```python
from build123d import *

# Parameters (mm, degrees)
SKETCH1_W           = 64.2
SKETCH1_H           = 22.5
SKETCH1_R           = 1.5
BOSS_EXTRUDE1_DEPTH = 18.8
SKETCH2_R           = 3
BOSS_EXTRUDE2_DEPTH = 18.4
SKETCH3_W           = 2.4
SKETCH3_H           = 2.701398926
SKETCH3_R           = 0.7
BOSS_EXTRUDE3_DEPTH = 1
FILLET1_R           = 2


with BuildPart() as part:
    # Sketch1 → Boss-Extrude1 (new body)
    with BuildSketch(Plane(origin=(0, 0, 0), x_dir=(1, 0, 0), z_dir=(0, 1, 0))):
        with Locations((32.1, 11.25)):
            Rectangle(SKETCH1_W, SKETCH1_H)
        with Locations(Location((32.4, 2.25, 0), (0, 0, 270))):
            Circle(SKETCH1_R, mode=Mode.SUBTRACT)
        with Locations(Location((32.4, 20.25, 0), (0, 0, 90))):
            Circle(SKETCH1_R, mode=Mode.SUBTRACT)
    extrude(amount=BOSS_EXTRUDE1_DEPTH)

    # Sketch2 → Boss-Extrude2 (add, symmetric)
    with BuildSketch(Plane(origin=(0, 9, 0), x_dir=(1, 0, 0), z_dir=(0, 1, 0))):
        with Locations(Location((53, 11.25, 0), (0, 0, 90))):
            Circle(SKETCH2_R)
    extrude(amount=BOSS_EXTRUDE2_DEPTH, both=True)

    # Sketch3 → Boss-Extrude3 (add, symmetric)
    with BuildSketch(Plane(origin=(0, 9, 0), x_dir=(1, 0, 0), z_dir=(0, 1, 0))):
        with Locations((65.4, 11.25)):
            Rectangle(SKETCH3_W, SKETCH3_H)
        with Locations(Location((65.4, 11.25, 0), (0, 0, 270))):
            Circle(SKETCH3_R, mode=Mode.SUBTRACT)
    extrude(amount=BOSS_EXTRUDE3_DEPTH, both=True)

    # Fillet1
    fillet1_edges = [part.edges().sort_by_distance(p)[0] for p in [
        (64.2, 9.4, -22.5),
        (64.2, 9.4, 0),
    ]]
    fillet(fillet1_edges, radius=FILLET1_R)


solid = part.part
```
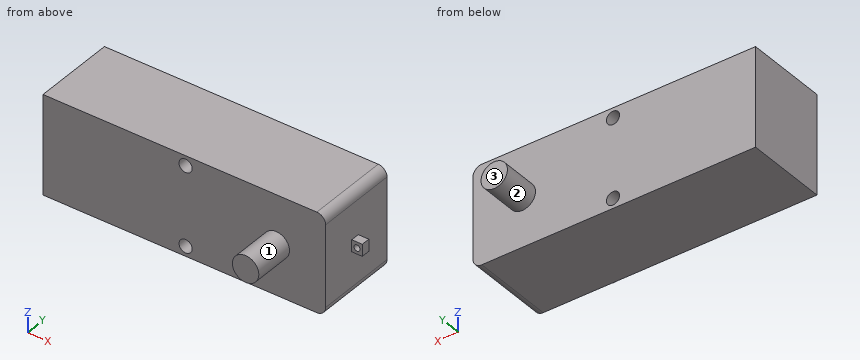
Could you check a few things on this model? Use its own coordinates, in mm. Face numbers are marked on the shaded views. A direction names the side the tool comes from. Round coordinates to 2 decimals unless told otherwise and drop trailing zeros. Loops run counter-clockwise (first coordinate to the right, second up) from the corner with the lowest first, then second, coordinate; pieces in that order, holes last. Notation, with made-up numbers: M 88.25,86.5 L 125.25,86.5 A12 cw 125.25,98.5 Z; hole C 19.25,-7.75 d11. An arc over 180 degrees is marked long. Put each result on its own line as item: value.
Q1. On a 3-axis mill with a long thin cutter (end or side, diameter ignored), from which of +Z, -Z, +X, -X, +Y, -Y can I reach the whole of each face in a straight line? I mean the marked faces 1, 2 and 3. Say none if no direction works.
Check result:
face 1: -Y
face 2: +Y
face 3: +Z, -Z, +X, -X, +Y
Q2. Imagine slicing it at C-C (y = 3). Write out the boundary of the cut face in (x, z).
Check result:
outline: M 0,-22.5 L 62.2,-22.5 A2 ccw 64.2,-20.5 L 64.2,-2 A2 ccw 62.2,0 L 0,0 Z; hole C 32.4,-20.25 d3; hole C 32.4,-2.25 d3
Q3. I need wall thicknesses on probe 1 along Z at (x, y) = (32.5, 12); probe 2 along X at (y, z) = (14.5, -2.25); probe 3 along Y at (x, z) = (19.5, -15.25). Which ranges of each line are inside material? Lowest first, please.
Check result:
probe 1: -22.5 to -21.75, -18.75 to -3.75, -0.75 to 0
probe 2: 0 to 30.9, 33.9 to 64.2
probe 3: 0 to 18.8
Q4. Imagine slicing it at B-B (z = -11.25). Write out the boundary of the cut face in (x, y).
Check result:
outline: M 0,0 L 50,0 L 50,-9.4 L 56,-9.4 L 56,0 L 64.2,0 L 64.2,8 L 64.7,8 L 64.7,10 L 64.2,10 L 64.2,18.8 L 56,18.8 L 56,27.4 L 50,27.4 L 50,18.8 L 0,18.8 Z; M 66.1,8 L 66.6,8 L 66.6,10 L 66.1,10 Z
Q5. For pin 1 (5 mm diameter, centred on x = 49.5, z = -5.5, fed in from -Y); pin 2 (11 mm diameter, centred on x = 19, z = -9.5, fed in from +Y); pin 3 (1.6 mm diameter, centred on x = 65.4, z = -11.25, fed in from -Y); pin 4 (1.8 mm diameter, centred on x = 32.4, z = -2.25, fed in from -Y), each with a flat end and sliding along its axis, tell me the tip position at first contact or that it passes through.
Check result:
pin 1: y = 0
pin 2: y = 18.8
pin 3: y = 8
pin 4: through
Q6. Imagine slicing it at A-A (x = 32.4). Write out the boundary of the cut face in (y, z), then the cut area to 3 significant figures.
Check result:
outline: M 0,-22.5 L 18.8,-22.5 L 18.8,-21.75 L 0,-21.75 Z; M 0,-18.75 L 18.8,-18.75 L 18.8,-3.75 L 0,-3.75 Z; M 0,-0.75 L 18.8,-0.75 L 18.8,0 L 0,0 Z
area: 310 mm2
Q7. Imagine slicing it at D-D (x = 53). Write out the boundary of the cut face in (y, z).
Check result:
outline: M -9.4,-14.25 L 0,-14.25 L 0,-22.5 L 18.8,-22.5 L 18.8,-14.25 L 27.4,-14.25 L 27.4,-8.25 L 18.8,-8.25 L 18.8,0 L 0,0 L 0,-8.25 L -9.4,-8.25 Z
